Geometry: final body of the model. Coordinates: model frame, mm. Face numbers are marked on the shaded views. A direction names the side the tool comes from. Give positions to 0.01 mm unless a question says otherwise; leave off trailing zeros. Order: outer loops, then holes, each group sorted by start corner. A loop starts at its lowest first (then second) coordinate and runs counter-clockwise, first axis right, second up. Notation, with made-up numbers: (0, 75.5) - (34, 75.5) arc R19 ccw to (34, 107.5) - close; hole circle Ø10 at (39, 10.5). An arc over 180 degrees is marked (long way). Put each result on its own line as item: value. Start each with the question number.
1. Set-up query: the marked faces 5, 6 and 7. Return all of +Z, -Z, +X, -X, +Y, -Y with unobstructed straight access to the full face (end or side cutting, diameter ignored); none if empty.
2. Section B-B on y = 19. Return the cut outline in (x, z).
3. Ray query, line 1 along Y through (x, z) = (15, 17); line 2 along Z through (x, y) = (11.5, -18.5); line 3 along X through (y, z) = (-0.5, -16). Return the intervals inside material, ascending. Write a range as from..to.
4. Mould query, pull axis Z, two halves, no side actions, for the marked faces 1, 2, 3 and 4. Classes: pulls with the +Z half, pulls with the -Z half, needs draft (parallel to the pull), parting line crosses it, or undercut.
5. First-contact query: P1, Ø5, axis at x = 13.5, y = 21.5, coming from the -Z side; P2, Ø6, axis at y = 0, z = -5.5, coming from the +X side; P3, Ø4, axis at x = 15, y = 19, coming from the +Z side. Flat tips, straight axial feed; report the tip coordinate or a pass-through.
6. Section A-A on x = 11.5. Return the cut outline in (y, z), plus the area to 3 significant figures.
7. Section C-C on x = 15.75. Count the separate pieces of the cut face and the enclosed holes in it, plus the area to 3 significant figures.
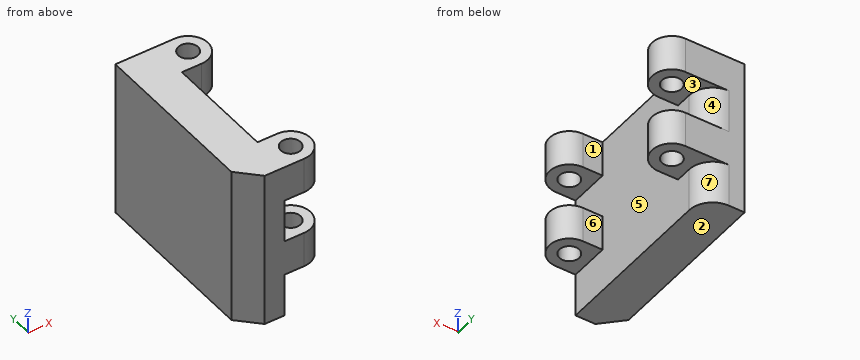
from build123d import *

# Parameters (mm, degrees)
SKETCH1_W           = 40
SKETCH1_H           = 48
BOSS_EXTRUDE1_DEPTH = 10
SKETCH6_R           = 2.5
BOSS_EXTRUDE2_DEPTH = 9
LPATTERN1_COUNT     = 2
LPATTERN1_PITCH     = 20
FILLET1_R           = 6
CHAMFER2_SIZE       = 5


with BuildPart() as part:
    # Sketch1 → Boss-Extrude1 (new body)
    with BuildSketch(Plane(origin=(0, 0, 0), x_dir=(0, 0, -1), z_dir=(1, 0, 0))):
        Rectangle(SKETCH1_W, SKETCH1_H)
    extrude(amount=BOSS_EXTRUDE1_DEPTH)

    # Sketch6 → Boss-Extrude2 (add)
    with BuildSketch(Plane.XY.offset(20)):
        with BuildLine():
            Line((5, 24), (15, 24))
            ThreePointArc((15, 24), (20, 19), (15, 14))
            Line((15, 14), (5, 14))
            ThreePointArc((5, 14), (0, 19), (5, 24))
        make_face()
        with Locations((15, 19)):
            Circle(SKETCH6_R, mode=Mode.SUBTRACT)
        with BuildLine():
            Line((5, -14), (15, -14))
            ThreePointArc((15, -14), (20, -19), (15, -24))
            Line((15, -24), (5, -24))
            ThreePointArc((5, -24), (0, -19), (5, -14))
        make_face()
        with Locations((15, -19)):
            Circle(SKETCH6_R, mode=Mode.SUBTRACT)
    boss_extrude2 = extrude(amount=-BOSS_EXTRUDE2_DEPTH)

    # LPattern1: Boss-Extrude2 ×2
    with Locations(*[(0, 0, -i * LPATTERN1_PITCH) for i in range(1, LPATTERN1_COUNT)]):
        add(boss_extrude2)

    # Fillet1
    fillet1_edges = [part.edges().sort_by_distance(p)[0] for p in [
        (10, 24, 5.5),
        (10, 24, -14.5),
    ]]
    fillet(fillet1_edges, radius=FILLET1_R)

    # Chamfer2
    chamfer2_edges = [part.edges().sort_by_distance(p)[0] for p in [
        (0, -24, 0),
    ]]
    chamfer(chamfer2_edges, length=CHAMFER2_SIZE)


solid = part.part
Resolved:
1. face 5: +X
1. face 6: +Z, -Z, +X
1. face 7: -Z, +X, +Y
2. outline: (0, -20) - (9.92, -20) - (9.92, -9) - (12.5, -9) - (12.5, 0) - (9.92, 0) - (9.92, 11) - (12.5, 11) - (12.5, 20) - (0, 20) - close; (17.5, -9) - (20, -9) - (20, 0) - (17.5, 0) - close; (17.5, 11) - (20, 11) - (20, 20) - (17.5, 20) - close
3. line 1: -24..-21.5, -16.5..-14, 14..16.5, 21.5..24
3. line 2: -9..0, 11..20
3. line 3: 0..10
4. face 1: needs draft
4. face 2: pulls with the -Z half
4. face 3: undercut
4. face 4: undercut
5. P1: z = -9
5. P2: x = 10
5. P3: through
6. outline: (-24, -9) - (-14, -9) - (-14, 0) - (-24, 0) - close; (-24, 11) - (-14, 11) - (-14, 20) - (-24, 20) - close; (14, -9) - (24, -9) - (24, 0) - (14, 0) - close; (14, 11) - (24, 11) - (24, 20) - (14, 20) - close
6. area: 360 mm^2
7. separate pieces: 8
7. enclosed holes: 0
7. area: 184 mm^2
